```python
from build123d import *

# Parameters (mm, degrees)
BOSS_EXTRUDE1_DEPTH      = 50
BOSS_EXTRUDE1_DEPTH_BACK = 50
SKETCH1_W                = 20
SKETCH1_H                = 20
CUT_EXTRUDE2_DEPTH       = 58.445626465


with BuildPart() as part:
    # Sketch1 → Boss-Extrude1 (new, two sides: drawn at the far end of the back side and taken through both)
    with BuildSketch(Plane(origin=(0, 0, 0), x_dir=(1, 0, 0), z_dir=(0, 1, 0)).offset(-BOSS_EXTRUDE1_DEPTH_BACK)):
        with Locations((10, -10)):
            Rectangle(SKETCH1_W, SKETCH1_H)
    extrude(amount=BOSS_EXTRUDE1_DEPTH + BOSS_EXTRUDE1_DEPTH_BACK)

    # Sketch3 → Cut-Extrude2 (cut, through all)
    with BuildSketch(Plane.ZY):
        Polygon((7.5, 40), (5, 40), (5, 37.171225458), (15, 37.171225458), (15, 40), (12.5, 40), (12.5, 50), (10, 50), (7.5, 50), align=None)
        Polygon((5, -37.171225458), (5, -40), (7.5, -40), (7.5, -50), (10, -50), (12.5, -50), (12.5, -40), (15, -40), (15, -37.171225458), align=None)
    extrude(amount=-CUT_EXTRUDE2_DEPTH, mode=Mode.SUBTRACT)


solid = part.part
```
For this review, take the finished solid that the model builds, in its own axes (mm). A direction names the side the tool comes from. Coordinates: 2 decimals unless noted, no trailing zeros. Write each loop counter-clockwise with the first axis right and the second up, starting at its lowest first coordinate (ties: lowest second). Pieces come first, ordered by that corner, then holes. Notation, with made-up numbers: (64, 69.25) - (77, 69.25) arc R23 ccw to (77, 90.25) - close; hole circle Ø3 at (33.25, -37). An arc over 180 degrees is marked (long way). Put each result on its own line as item: value.
1. Add section A-A, the plane x = 11.25. Give the boundary of the cut face in (y, z).
Values found:
outline: (-50, 0) - (50, 0) - (50, 7.5) - (40, 7.5) - (40, 5) - (37.17, 5) - (37.17, 15) - (40, 15) - (40, 12.5) - (50, 12.5) - (50, 20) - (-50, 20) - (-50, 12.5) - (-40, 12.5) - (-40, 15) - (-37.17, 15) - (-37.17, 5) - (-40, 5) - (-40, 7.5) - (-50, 7.5) - close
2. Machinability: for faces 1 (the flat face through (10, 45, 12.5)), 2 (the flat face through (10, 50, 16)), 3 (the flat face through (10, -40, 6)), 4 (the flat face through (0, -1, 10)), 5 (the flat face through (10, -45, 7.5)), which of the approach directions +Z, -Z, +X, -X, +Y, -Y give a long, thin tool a straight path to every point of the face, cutting with its end or side? Answer none if there is none.
Values found:
face 1: +X, -X, +Y
face 2: +Z, -Z, +X, -X, +Y
face 3: +X, -X
face 4: +Z, -Z, -X, +Y, -Y
face 5: +X, -X, -Y
3. Add section B-B, the plane z = 8.75. Give the boundary of the cut face in (x, y).
Values found:
outline: (0, -37.17) - (20, -37.17) - (20, 37.17) - (0, 37.17) - close
4. Wall thickness on probe 1 along Z at (x, y) = (14, 41.5); probe 2 along Y at (x, z) = (2, 5.5); probe 3 along Y at (x, z) = (19.25, 12): over which ranges is each line inside the solid? List them lowest first.
Values found:
probe 1: 0 to 7.5, 12.5 to 20
probe 2: -50 to -40, -37.17 to 37.17, 40 to 50
probe 3: -37.17 to 37.17
5. Mouldability with a two-part tool opening along Y and no side actions: class faces 6 (the flat face through (10, -50, 16)), 7 (the flat face through (10, 40, 6)), 8 (the flat face through (10, 39, 5)), 9 (the flat face through (20, -1, 10)) as released by +Y, released by -Y, zero draft, split by the parting line, or undercut.
Values found:
face 6: released by -Y
face 7: undercut
face 8: undercut
face 9: zero draft
